Check sheet for the modelled part. Datum: model origin and axes. Units: mm. A direction names the side the tool comes from. Coordinates: 2 decimals unless noted, no trailing zeros. Write each loop counter-clockwise with the first axis right and the second up, starting at its lowest first coordinate (ties: lowest second). Pieces come first, ordered by that corner, then holes. Notation, with made-up numbers: (38.25, -25.75) -> (58.25, -25.75) arc R25 cw to (58.25, 13.25) -> close; hole circle Ø9 at (31.5, 33). An arc over 180 degrees is marked (long way). One line per item, written item: value. Start each with the question number.
1) Sectioned sample at C-C on z = 0.9. Give the number of separate pieces and of enclosed holes in the cut face, plus the area to 3 significant figures.
2) Scan lines: line 1 along Y through (x, z) = (0, 1.4); line 2 along Y through (x, z) = (-1, 1.05); line 3 along X through (y, z) = (-10, 2.65). Record each from-to range of solid material in increasing order. Write a range as [from, to].
3) Sectioned sample at B-B on y = -6. Enter the section's corners in (x, z), plus the area to 3 significant figures.
4) Set-up check for faces 3 (the flat face through (18.158, 0, 1)), 4 (the cylindrical face through (29.194, 13.996, 2.282)), 5 (the cylindrical face through (-15.484, 17.035, 3.514)): record each of +Z, -Z, +X, -X, +Y, -Y from which the full face is reachable in a straight line by a thin tool's end or side.
5) Gauge pin test, flat ends, axial feed: P1, Ø1.8, axis at x = -8.84, y = -8.84, coming from the -Z side; P2, Ø23.5, axis at x = 0, y = 0, coming from the +Z side; P3, Ø1.5, axis at y = 7, z = 1, coming from the +X side; P4, Ø1.2, axis at y = -14.5, z = 1.5, coming from the +X side. Record the tip position at first contact, or that the pin passes through.
6) Sectioned sample at A-A on y = 0. Enter the section's corners in (x, z), plus the area to 3 significant figures.
7) Draft check along Y on faces 1 (the flat face through (-14.28, 2.26, 0.99)), 2 (the flat face through (0, 22.5, 2)). Enter one of: +Y half, -Y half, draft (parallel to the pull), parting line (faces both ways), or undercut.
```python
from build123d import *

# Parameters (mm, degrees)
SKETCH_1_W          = 60
SKETCH_1_H          = 45
SKETCH_1_R          = 1.5
SKETCH_1_R_2        = 9
EXTRUDE_1_DEPTH     = 4.5
CUT_EXTRUDE_1_DEPTH = 2
FILLET_1_R          = 5
SKETCH_4_R          = 1.8
CUT_EXTRUDE_2_DEPTH = 4.5
CUT_EXTRUDE_3_DEPTH = 2.5
CUT_EXTRUDE_4_DEPTH = 4.5
FILLET_2_R          = 6


with BuildPart() as part:
    # 草图1 → 凸台-拉伸1 (new body)
    with BuildSketch(Plane.XY):
        Rectangle(SKETCH_1_W, SKETCH_1_H)
        with Locations((8.838834765, 8.838834765)):
            Circle(SKETCH_1_R, mode=Mode.SUBTRACT)
        Circle(SKETCH_1_R_2, mode=Mode.SUBTRACT)
        with Locations((8.838834765, -8.838834765)):
            Circle(SKETCH_1_R, mode=Mode.SUBTRACT)
        with Locations((-8.838834765, -8.838834765)):
            Circle(SKETCH_1_R, mode=Mode.SUBTRACT)
        with Locations((-8.838834765, 8.838834765)):
            Circle(SKETCH_1_R, mode=Mode.SUBTRACT)
        with Locations((0, -15.56)):
            Circle(SKETCH_1_R, mode=Mode.SUBTRACT)
        with Locations((-15.56, 0)):
            Circle(SKETCH_1_R, mode=Mode.SUBTRACT)
        with Locations((0, 15.56)):
            Circle(SKETCH_1_R, mode=Mode.SUBTRACT)
        with Locations((15.56, 0)):
            Circle(SKETCH_1_R, mode=Mode.SUBTRACT)
        with Locations((-25, 17.5)):
            Circle(SKETCH_1_R, mode=Mode.SUBTRACT)
        with Locations((25, 17.5)):
            Circle(SKETCH_1_R, mode=Mode.SUBTRACT)
        with Locations((25, -17.5)):
            Circle(SKETCH_1_R, mode=Mode.SUBTRACT)
        with Locations((-25, -17.5)):
            Circle(SKETCH_1_R, mode=Mode.SUBTRACT)
    extrude(amount=EXTRUDE_1_DEPTH)

    # 草图2 → 切除-拉伸1 (cut)
    with BuildSketch(Plane(origin=(0, 0, 0), x_dir=(-1, 0, 0), z_dir=(0, 0, -1))):
        Polygon((-1.5, -12.961923789), (-3, -15.56), (-1.5, -18.158076211), (1.5, -18.158076211), (3, -15.56), (1.5, -12.961923789), align=None)
        Polygon((12.961923789, -1.5), (15.56, -3), (18.158076211, -1.5), (18.158076211, 1.5), (15.56, 3), (12.961923789, 1.5), align=None)
        Polygon((-12.961923789, 1.5), (-15.56, 3), (-18.158076211, 1.5), (-18.158076211, -1.5), (-15.56, -3), (-12.961923789, -1.5), align=None)
        Polygon((1.5, 12.961923789), (3, 15.56), (1.5, 18.158076211), (-1.5, 18.158076211), (-3, 15.56), (-1.5, 12.961923789), align=None)
    extrude(amount=-CUT_EXTRUDE_1_DEPTH, mode=Mode.SUBTRACT)

    # 圆角1
    fillet_1_edges = [part.edges().sort_by_distance(p)[0] for p in [
        (30, -22.5, 2.25),
        (-30, -22.5, 2.25),
        (-30, 22.5, 2.25),
        (30, 22.5, 2.25),
    ]]
    fillet(fillet_1_edges, radius=FILLET_1_R)

    # 草图4 → 切除-拉伸2 (cut)
    with BuildSketch(Plane.XY.offset(4.5)):
        with Locations((-15.25, 15.25)):
            Circle(SKETCH_4_R)
        with Locations((15.25, 15.25)):
            Circle(SKETCH_4_R)
        with Locations((15.25, -15.25)):
            Circle(SKETCH_4_R)
        with Locations((-15.25, -15.25)):
            Circle(SKETCH_4_R)
    extrude(amount=-CUT_EXTRUDE_2_DEPTH, mode=Mode.SUBTRACT)

    # 草图5 → 切除-拉伸3 (cut)
    with BuildSketch(Plane(origin=(0, 0, 0), x_dir=(-1, 0, 0), z_dir=(0, 0, -1))):
        Polygon((12.651923789, 13.75), (15.25, 12.25), (17.848076211, 13.75), (17.848076211, 16.75), (15.25, 18.25), (12.651923789, 16.75), align=None)
        Polygon((-13.75, 12.651923789), (-12.25, 15.25), (-13.75, 17.848076211), (-16.75, 17.848076211), (-18.25, 15.25), (-16.75, 12.651923789), align=None)
        Polygon((13.75, -12.651923789), (12.25, -15.25), (13.75, -17.848076211), (16.75, -17.848076211), (18.25, -15.25), (16.75, -12.651923789), align=None)
        Polygon((-12.651923789, -13.75), (-15.25, -12.25), (-17.848076211, -13.75), (-17.848076211, -16.75), (-15.25, -18.25), (-12.651923789, -16.75), align=None)
    extrude(amount=-CUT_EXTRUDE_3_DEPTH, mode=Mode.SUBTRACT)

    # 草图6 → 切除-拉伸4 (cut)
    with BuildSketch(Plane(origin=(0, 0, 0), x_dir=(-1, 0, 0), z_dir=(0, 0, -1))):
        with BuildLine():
            Line((-30, 13), (-30, -13))
            ThreePointArc((-30, -13), (-20, 0), (-30, 13))
        make_face()
        with BuildLine():
            Line((30, -13), (30, 13))
            ThreePointArc((30, 13), (20, 0), (30, -13))
        make_face()
    extrude(amount=-CUT_EXTRUDE_4_DEPTH, mode=Mode.SUBTRACT)

    # 圆角2
    fillet_2_edges = [part.edges().sort_by_distance(p)[0] for p in [
        (30, -13, 2.25),
        (30, 13, 2.25),
        (-30, 13, 2.25),
        (-30, -13, 2.25),
    ]]
    fillet(fillet_2_edges, radius=FILLET_2_R)


solid = part.part
```
Answers:
1. separate pieces: 1
1. enclosed holes: 17
1. area: 1,790 mm2
2. line 1: y = [-22.5, -18.16], [-12.96, -9], [9, 12.96], [18.16, 22.5]
2. line 2: y = [-22.5, -18.16], [-12.96, -8.94], [8.94, 12.96], [18.16, 22.5]
2. line 3: x = [-24.46, -9.79], [-7.89, 7.89], [9.79, 24.46]
3. outline: (-21.41, 0) -> (-6.71, 0) -> (-6.71, 4.5) -> (-21.41, 4.5) -> close; (6.71, 0) -> (21.41, 0) -> (21.41, 4.5) -> (6.71, 4.5) -> close
3. area: 132 mm2
4. face 3: -Z
4. face 4: +Z, -Z, +X
4. face 5: +Z, -Z
5. P1: passes through
5. P2: stops at z = 4.5
5. P3: stops at x = 22.46
5. P4: stops at x = 29.69
6. outline: (-20, 0) -> (-18.16, 0) -> (-18.16, 2) -> (-17.06, 2) -> (-17.06, 4.5) -> (-20, 4.5) -> close; (-14.06, 2) -> (-12.96, 2) -> (-12.96, 0) -> (-9, 0) -> (-9, 4.5) -> (-14.06, 4.5) -> close; (9, 0) -> (12.96, 0) -> (12.96, 2) -> (14.06, 2) -> (14.06, 4.5) -> (9, 4.5) -> close; (17.06, 2) -> (18.16, 2) -> (18.16, 0) -> (20, 0) -> (20, 4.5) -> (17.06, 4.5) -> close
6. area: 63.2 mm2
7. face 1: undercut
7. face 2: +Y half
